Autodesk Inventor part; units mm, degrees
ref_plane "YZ Plane" through (0, 0, 0) normal (1, 0, 0) x (0, 1, 0)
ref_plane "XZ Plane" through (0, 0, 0) normal (0, 1, 0) x (-1, 0, 0)
ref_plane "XY Plane" through (0, 0, 0) normal (0, 0, 1) x (1, 0, 0)
sketch "Sketch1" plane through (0, 0, 0) normal (0, 1, 0) x (-1, 0, 0)
  line L0 (6.35, -3.6662) -> (0, -7.3323)
  line L1 (0, -7.3323) -> (-6.35, -3.6662)
  line L2 (-6.35, -3.6662) -> (-6.35, 3.6662)
  line L3 (-6.35, 3.6662) -> (0, 7.3323)
  line L4 (0, 7.3323) -> (6.35, 3.6662)
  line L5 (6.35, 3.6662) -> (6.35, -3.6662)
  point P0 (0, 0)
  point P1 (0, 0)
  point P2 (0, 0)
  dimension "d0" = 12.7
extrude "Extrusion1" add sketch "Sketch1" along normal blind 126.4412
sketch "Sketch2" plane through (0, 126.4412, 0) normal (0, 1, 0) x (1, 0, 0)
  point P0 (0, 0)
  point P1 (0, 0)
hole "Hole1" at (0, 126.4412, 0) direction (0, -1, 0) diameter 4.9784 depth 25.4
sketch "Sketch3" plane through (0, 0, 0) normal (0, -1, 0) x (1, 0, 0)
  point P0 (0, 0)
  point P1 (0, 0)
hole "Hole2" at (0, 0, 0) direction (0, 1, 0) diameter 4.9784 depth 25.4
properties part number "ELEV_039_HEXSHAFT3" material "Aluminum 6061"
Could you check a few things on this model? Use its own coordinates, in mm. A direction names the side the tool comes from. Coordinates: 2 decimals unless noted, no trailing zeros. Write each loop counter-clockwise with the first axis right and the second up, starting at its lowest first coordinate (ties: lowest second). Pieces come first, ordered by that corner, then holes. Notation, with made-up numbers: (10.25, 55) -> (14.25, 55) arc R27 ccw to (14.25, 90) -> close; hole circle Ø3 at (38, 9.5). An arc over 180 degrees is marked (long way). Write item = value, one per line. Start each with the question number.
(1) I want a section at D-D (x = -4.5). Please give me the cut outline in (y, z), plus the area to 3 significant figures.
(2) I want a section at A-A (y = 14.5). Please give me the cut outline in (x, z).
(3) I need wall thicknesses on line 1 (Z direction, x = 0, y = 17.75); line 2 (X direction, y = 110.75, z = 0); line 3 (Y direction, x = -2, z = 0.5). Which ranges of each line are inside material? Lowest first, please. Write a range as [from, to].
(4) Will these pins go through, and if not, where does the flat tip stop? pin 1 (1.5 mm diameter, centred on x = -1, z = 0.5, fed in from +Y); pin 2 (2 mm diameter, centred on x = -4, y = 58.5, fed in from +Z); pin 3 (1.5 mm diameter, centred on y = 31, z = 5.5, fed in from -X).
(5) Which directions (+Z, -Z, +X, -X, +Y, -Y) give clear straight access to the entire face, cutting with the end or side of a thin tool? Please do faces 1 (the face through (6.35, 62, 0)), 2 (the face through (0, 25.4, 0)), 3 (the face through (0, 101.041, 0)).
(6) I want a section at C-C (y = 78.5). Please give me the cut outline in (x, z).
(7) We'd pull the mould along Z, two halves only. Please class faces 4 (the face through (-0.748, 12.878, -2.374)), 5 (the face through (3.219, 62.336, 5.474)), 6 (the face through (3.131, 62.336, -5.525)), 7 (the face through (-6.35, 62, 0)): released by +Z, released by -Z, zero draft, split by the parting line, or undercut.
(8) I want a section at B-B (z = 0). Please give me the cut outline in (x, y).
Result set:
q1.outline = (0, -4.73) -> (126.44, -4.73) -> (126.44, 4.73) -> (0, 4.73) -> close
q1.area = 1,200 mm2
q2.outline = (-6.35, -3.67) -> (0, -7.33) -> (6.35, -3.67) -> (6.35, 3.67) -> (0, 7.33) -> (-6.35, 3.67) -> close; hole circle Ø4.98 at (0, 0)
q3.line_1 = [-7.33, -2.49], [2.49, 7.33]
q3.line_2 = [-6.35, -2.49], [2.49, 6.35]
q3.line_3 = [25.4, 101.04]
q4.pin_1 = 101.04
q4.pin_2 = 5.6
q4.pin_3 = -4.47
q5.face_1 = +Z, -Z, +X, +Y, -Y
q5.face_2 = -Y
q5.face_3 = +Y
q6.outline = (-6.35, -3.67) -> (0, -7.33) -> (6.35, -3.67) -> (6.35, 3.67) -> (0, 7.33) -> (-6.35, 3.67) -> close
q7.face_4 = undercut
q7.face_5 = released by +Z
q7.face_6 = released by -Z
q7.face_7 = zero draft
q8.outline = (-6.35, 0) -> (-2.49, 0) -> (-2.49, 25.4) -> (2.49, 25.4) -> (2.49, 0) -> (6.35, 0) -> (6.35, 126.44) -> (2.49, 126.44) -> (2.49, 101.04) -> (-2.49, 101.04) -> (-2.49, 126.44) -> (-6.35, 126.44) -> close
